```python
from build123d import *
from OCP.BRepFilletAPI import BRepFilletAPI_MakeChamfer

# Parameters (mm, degrees)
SKETCH_1_W       = 40.5
SKETCH_1_H       = 19.8
BODY_DEPTH       = 36.5
CHAMFER_1_SIZE   = 2.2
CHAMFER_1_SIZE2  = 1.4
FILLET_1_R       = 0.5
MOUNT_DEPTH      = 2.5
FILLET_3_R       = 1
EXTRUDE_3_DEPTH  = 0.5
EXTRUDE_4_DEPTH  = 2
SKETCH_5_W       = 10.8
SKETCH_5_H       = 15.84
EXTRUDE_5_DEPTH  = 0.2
SKETCH_6_R       = 6.6
EXTRUDE_6_DEPTH  = 1.2
SKETCH_7_R       = 5.35
EXTRUDE_7_DEPTH  = 0.5
SKETCH_8_R       = 2.6
SHAFT_HOLE_DEPTH = 10
FILLET_2_R       = 0.5
SKETCH_11_R      = 0.75
EXTRUDE_10_DEPTH = 8


with BuildPart() as part:
    # Эскиз1 → Body (new body)
    with BuildSketch(Plane(origin=(0, 0, 0), x_dir=(1, 0, 0), z_dir=(0, 1, 0))):
        Rectangle(SKETCH_1_W, SKETCH_1_H)
    extrude(amount=BODY_DEPTH)

    # Фаска1: one chamfer whose edges measure the first distance from different faces: ONE call of the kernel's chamfer builder (chamfer() names one face for all edges)
    chamfer_1_edges_1 = [part.edges().sort_by_distance(p)[0] for p in [
        (20.25, 36.5, 0),
    ]]
    chamfer_1_side_1 = [part.faces().sort_by_distance(p)[0] for p in [
        (20.25, 18.25, 0),
    ]]
    chamfer_1_edges_2 = [part.edges().sort_by_distance(p)[0] for p in [
        (0, 36.5, -9.9),
    ]]
    chamfer_1_side_2 = [part.faces().sort_by_distance(p)[0] for p in [
        (0, 18.25, -9.9),
    ]]
    chamfer_1_edges_3 = [part.edges().sort_by_distance(p)[0] for p in [
        (-20.25, 36.5, 0),
    ]]
    chamfer_1_side_3 = [part.faces().sort_by_distance(p)[0] for p in [
        (-20.25, 18.25, 0),
    ]]
    chamfer_1_edges_4 = [part.edges().sort_by_distance(p)[0] for p in [
        (0, 36.5, 9.9),
    ]]
    chamfer_1_side_4 = [part.faces().sort_by_distance(p)[0] for p in [
        (0, 18.25, 9.9),
    ]]
    chamfer_1 = BRepFilletAPI_MakeChamfer(part.part.solid().wrapped)
    for e in chamfer_1_edges_1:
        chamfer_1.Add(CHAMFER_1_SIZE, CHAMFER_1_SIZE2, e.wrapped, chamfer_1_side_1[0].wrapped)  # the first distance lies on this face
    for e in chamfer_1_edges_2:
        chamfer_1.Add(CHAMFER_1_SIZE, CHAMFER_1_SIZE2, e.wrapped, chamfer_1_side_2[0].wrapped)  # the first distance lies on this face
    for e in chamfer_1_edges_3:
        chamfer_1.Add(CHAMFER_1_SIZE, CHAMFER_1_SIZE2, e.wrapped, chamfer_1_side_3[0].wrapped)  # the first distance lies on this face
    for e in chamfer_1_edges_4:
        chamfer_1.Add(CHAMFER_1_SIZE, CHAMFER_1_SIZE2, e.wrapped, chamfer_1_side_4[0].wrapped)  # the first distance lies on this face
    add(Compound.cast(chamfer_1.Shape()), mode=Mode.REPLACE)

    # Скругление1
    # the kernel refuses this fillet: 0.5 mm, written as the material it takes off along each edge
    with BuildSketch(Plane(origin=(-20.25, -1.25, 9.9), x_dir=(1, 0, 0), z_dir=(0, 1, 0)), Plane(origin=(-20.25, -1.25, -9.9), x_dir=(0, 0, 1), z_dir=(0, 1, 0))) as fillet_1_piece_1:
        with BuildLine():
            CenterArc((FILLET_1_R, FILLET_1_R), FILLET_1_R, 180, 90)
            Line((0, FILLET_1_R), (0, 0))
            Line((0, 0), (FILLET_1_R, 0))
        make_face()
    extrude(amount=36.8, mode=Mode.SUBTRACT)
    with BuildSketch(Plane(origin=(20.25, -1.25, -9.9), x_dir=(0, 0, 1), z_dir=(0, 1, 0)), Plane(origin=(20.25, -1.25, 9.9), x_dir=(-1, 0, 0), z_dir=(0, 1, 0))) as fillet_1_piece_2:
        with BuildLine():
            CenterArc((FILLET_1_R, -FILLET_1_R), FILLET_1_R, 90, 90)
            Line((0, -FILLET_1_R), (0, 0))
            Line((0, 0), (FILLET_1_R, 0))
        make_face()
    extrude(amount=36.8, mode=Mode.SUBTRACT)
    with BuildSketch(Plane(origin=(20.689497717, 33.609360731, -10.339497717), x_dir=(0.25395078633508533, -0.3990655213836877, 0.8810537485094523), z_dir=(-0.47301616487963943, 0.7433111162394352, 0.47301616487964004)), Plane(origin=(20.689497717, 33.609360731, 10.339497717), x_dir=(-0.8810537485094526, -0.39906552138369156, 0.25395078633507817), z_dir=(-0.47301616487963943, 0.7433111162394352, -0.47301616487964004))) as fillet_1_piece_3:
        with BuildLine():
            CenterArc((FILLET_1_R * 0.743311116239, -FILLET_1_R), FILLET_1_R, 90, 73.247664886)
            Line((-FILLET_1_R * 0.21424849821, -FILLET_1_R * 0.711764705882), (0, 0))
            Line((0, 0), (FILLET_1_R * 0.743311116239, 0))
        make_face()
    extrude(amount=4.818007508, mode=Mode.SUBTRACT)
    with BuildSketch(Plane(origin=(-20.689497717, 33.609360731, -10.339497717), x_dir=(-0.25395078633507856, -0.3990655213836921, 0.8810537485094524), z_dir=(0.47301616487963943, 0.7433111162394352, 0.47301616487964004)), Plane(origin=(-20.689497717, 33.609360731, 10.339497717), x_dir=(0.8810537485094527, -0.3990655213836916, 0.25395078633507817), z_dir=(0.47301616487963943, 0.7433111162394352, -0.47301616487964004))) as fillet_1_piece_4:
        with BuildLine():
            CenterArc((FILLET_1_R * 0.743311116239, FILLET_1_R), FILLET_1_R, 196.752335114, 73.247664886)
            Line((-FILLET_1_R * 0.21424849821, FILLET_1_R * 0.711764705882), (0, 0))
            Line((0, 0), (FILLET_1_R * 0.743311116239, 0))
        make_face()
    extrude(amount=4.818007508, mode=Mode.SUBTRACT)

    # Эскиз2 → Mount (add)
    with BuildSketch(Plane(origin=(0, 6.2, 0), x_dir=(-1, 0, 0), z_dir=(0, -1, 0))):
        with BuildLine():
            Line((-26.85, 9.472835762), (26.85, 9.472835762))
            Line((26.85, 9.472835762), (26.85, 6.069767442))
            Line((26.85, 6.069767442), (26.229418506, 6.069767442))
            ThreePointArc((26.229418506, 6.069767442), (22, 5), (26.229418506, 3.930232558))
            Line((26.229418506, 3.930232558), (26.85, 3.930232558))
            Line((26.85, 3.930232558), (26.85, -3.930232558))
            Line((26.85, -3.930232558), (26.229418506, -3.930232558))
            ThreePointArc((26.229418506, -3.930232558), (22, -5), (26.229418506, -6.069767442))
            Line((26.229418506, -6.069767442), (26.85, -6.069767442))
            Line((26.85, -6.069767442), (26.85, -9.4))
            Line((26.85, -9.4), (-26.85, -9.4))
            Line((-26.85, -9.4), (-26.85, -6.069767442))
            Line((-26.85, -6.069767442), (-26.229418506, -6.069767442))
            ThreePointArc((-26.229418506, -6.069767442), (-22, -5), (-26.229418506, -3.930232558))
            Line((-26.229418506, -3.930232558), (-26.85, -3.930232558))
            Line((-26.85, -3.930232558), (-26.85, 3.930232558))
            Line((-26.85, 3.930232558), (-26.229418506, 3.930232558))
            ThreePointArc((-26.229418506, 3.930232558), (-22, 5), (-26.229418506, 6.069767442))
            Line((-26.229418506, 6.069767442), (-26.85, 6.069767442))
            Line((-26.85, 6.069767442), (-26.85, 9.472835762))
        make_face()
    extrude(amount=-MOUNT_DEPTH)

    # Скругление3
    fillet_3_edges = [part.edges().sort_by_distance(p)[0] for p in [
        (-26.85, 7.45, 9.4),
        (26.85, 7.45, 9.4),
        (26.85, 7.45, -9.472835762),
        (-26.85, 7.45, -9.472835762),
    ]]
    fillet(fillet_3_edges, radius=FILLET_3_R)

    # Эскиз3 → Бобышка-Вытянуть3 (add, symmetric)
    with BuildSketch(Plane.XY):
        Polygon((-26.85, 6.2), (-20.25, 6.2), (-20.25, 5.2), align=None)
        Polygon((20.25, 5.2), (26.85, 6.2), (20.25, 6.2), align=None)
    extrude(amount=EXTRUDE_3_DEPTH, both=True)

    # Эскиз4 → Бобышка-Вытянуть4 (add)
    with BuildSketch(Plane.XZ):
        with BuildLine():
            Line((-13.452560024, -8.92), (-13.452560024, -4.6))
            ThreePointArc((-13.452560024, -4.6), (-16.49296823, 0), (-13.452560024, 4.6))
            Line((-13.452560024, 4.6), (-13.452560024, 8.92))
            Line((-13.452560024, 8.92), (6.568139057, 8.92))
            ThreePointArc((6.568139057, 8.92), (19.9, 0), (6.568139057, -8.92))
            Line((6.568139057, -8.92), (-13.452560024, -8.92))
        make_face()
    extrude(amount=EXTRUDE_4_DEPTH)

    # Эскиз5 → Бобышка-Вытянуть5 (add)
    with BuildSketch(Plane.XZ.offset(2)):
        with BuildLine():
            Line((-13.452560024, 8.92), (-0.652560024, 8.92))
            Line((-0.652560024, 8.92), (-0.652560024, 2))
            ThreePointArc((-0.652560024, 2), (1.347439976, 0), (-0.652560024, -2))
            Line((-0.652560024, -2), (-0.652560024, -8.92))
            Line((-0.652560024, -8.92), (-13.452560024, -8.92))
            Line((-13.452560024, -8.92), (-13.452560024, 8.92))
        make_face()
        with Locations((-7.052560024, 0)):
            Rectangle(SKETCH_5_W, SKETCH_5_H, mode=Mode.SUBTRACT)
    extrude(amount=EXTRUDE_5_DEPTH)

    # Эскиз6 → Бобышка-Вытянуть6 (add)
    with BuildSketch(Plane.XZ.offset(2)):
        with Locations(Location((10.25, 0, 0), (0, 0, 270))):
            Circle(SKETCH_6_R)
    extrude(amount=EXTRUDE_6_DEPTH)

    # Эскиз7 → Бобышка-Вытянуть7 (add)
    with BuildSketch(Plane.XZ.offset(3.2)):
        with Locations(Location((10.25, 0, 0), (0, 0, 270))):
            Circle(SKETCH_7_R)
    extrude(amount=EXTRUDE_7_DEPTH)

    # Эскиз8 → Shaft hole (cut)
    with BuildSketch(Plane.XZ.offset(3.7)):
        with Locations(Location((10.25, 0, 0), (0, 0, 270))):
            Circle(SKETCH_8_R)
    extrude(amount=-SHAFT_HOLE_DEPTH, mode=Mode.SUBTRACT)

    # Скругление2
    fillet_2_edges = [part.edges().sort_by_distance(p)[0] for p in [
        (-13.452560024, -1.1, 8.92),
        (-0.652560024, -2.1, 2),
        (-0.652560024, -2.1, -2),
        (-0.652560024, -2.1, 8.92),
        (-0.652560024, -2.1, -8.92),
        (-13.452560024, -1.1, -8.92),
        (-1.652560024, -2.1, 7.92),
        (-1.652560024, -2.1, -7.92),
        (-12.452560024, -2.1, 7.92),
        (-12.452560024, -2.1, -7.92),
    ]]
    fillet(fillet_2_edges, radius=FILLET_2_R)

    # Эскиз10 → Rubber section 0
    with BuildSketch(Plane(origin=(25.25, 0, 0), x_dir=(0, 0, -1), z_dir=(1, 0, 0))):
        with BuildLine():
            Line((-2.5, 29.75), (2.5, 29.75))
            Line((2.5, 29.75), (2.5, 32.55))
            Line((2.5, 32.55), (-2.5, 32.55))
            Line((-2.5, 32.55), (-2.5, 29.75))
        make_face()
    # Эскиз9 → Rubber section 1
    with BuildSketch(Plane(origin=(20.25, 0, 0), x_dir=(0, 0, -1), z_dir=(1, 0, 0))):
        with BuildLine():
            Line((-3.4, 33.3), (3.4, 33.3))
            Line((3.4, 33.3), (3.4, 29))
            Line((3.4, 29), (-3.4, 29))
            Line((-3.4, 29), (-3.4, 33.3))
        make_face()
    loft()

    # Эскиз11 → Бобышка-Вытянуть10 (add)
    with BuildSketch(Plane(origin=(25.25, 0, 0), x_dir=(0, 0, -1), z_dir=(1, 0, 0))):
        with Locations(Location((0, 31.150503064, 0), (0, 0, 180))):
            Circle(SKETCH_11_R)
        with Locations(Location((1.509999917, 31.15000331, 0), (0, 0, 180))):
            Circle(SKETCH_11_R)
        with Locations(Location((-1.509999915, 31.149996646, 0), (0, 0, 180))):
            Circle(SKETCH_11_R)
    extrude(amount=EXTRUDE_10_DEPTH)


solid = part.part
```
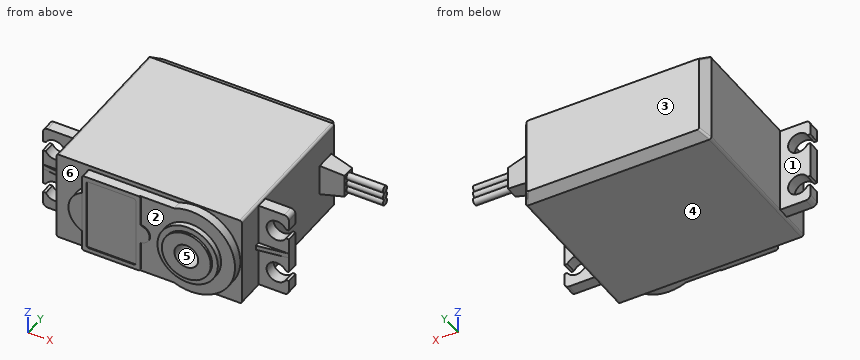
CAD build for the part. Positions are in the model's coordinates, mm. Face numbers are marked on the shaded views. A direction names the side the tool comes from. Coordinates: 2 decimals unless noted, no trailing zeros. Loops run counter-clockwise (first coordinate to the right, second up) from the corner with the lowest first, then second, coordinate; pieces in that order, holes last. Notation, with made-up numbers: (53, 37) - (98, 37) arc R24 ccw to (98, 76) - close; hole circle Ø4 at (24, 14.5). An arc over 180 degrees is marked (long way). Return JSON: item names as keys, results as strings.
1. Band-saw the part on D-D (y = 16). Give the cut face in (x, z).
Result:
{"outline": "(-20.25, -9.4) arc R0.5 ccw to (-19.75, -9.9) - (19.75, -9.9) arc R0.5 ccw to (20.25, -9.4) - (20.25, 9.4) arc R0.5 ccw to (19.75, 9.9) - (-19.75, 9.9) arc R0.5 ccw to (-20.25, 9.4) - close"}
2. Band-saw the part on A-A (x = -24.25). Give the cut face in (y, z), and give its area (3 significant figures).
Result:
{"outline": "(5.81, -0.5) - (6.2, -0.5) - (6.2, -2.75) - (8.7, -2.75) - (8.7, 2.75) - (6.2, 2.75) - (6.2, 0.5) - (5.81, 0.5) - close; (6.2, -9.47) - (8.7, -9.47) - (8.7, -7.25) - (6.2, -7.25) - close; (6.2, 7.25) - (8.7, 7.25) - (8.7, 9.4) - (6.2, 9.4) - close", "area": "25.1 mm2"}
3. 3-axis set-ups, long thin cutter, end or side, ignore diameter. For the marked faces 1, 2 and 3: which of +Z, -Z, +X, -X, +Y, -Y reach the whole face in a straight line?
Result:
{"face 1": "+Z, -Z, -X, +Y", "face 2": "-Y", "face 3": "+Z, -Z, +X, -X, +Y"}
4. Drop flat-ended pins along their axis: pin 1 (0.7 mm diameter, centred on x = -23.5, y = 7, fed in from -Z); pin 2 (8 mm diameter, centred on x = -16, z = -0.5, fed in from -Y); pin 3 (0.5 mm diameter, centred on x = -26.5, y = 8, fed in from -Z). Give the stop position or say it passes through.
Result:
{"pin 1": "stops at z = -9.47", "pin 2": "stops at y = -2.2", "pin 3": "stops at z = -9.39"}
5. Band-saw the part on C-C (x = 10.25). Give the cut face in (y, z).
Result:
{"outline": "(-3.7, -5.35) - (-3.2, -5.35) - (-3.2, -6.6) - (-2, -6.6) - (-2, -9.65) - (0, -9.65) - (0, -9.9) - (34.3, -9.9) - (36.5, -8.5) - (36.5, 8.5) - (34.3, 9.9) - (0, 9.9) - (0, 9.65) - (-2, 9.65) - (-2, 6.6) - (-3.2, 6.6) - (-3.2, 5.35) - (-3.7, 5.35) - (-3.7, 2.6) - (6.3, 2.6) - (6.3, -2.6) - (-3.7, -2.6) - close"}
6. Probe L1, parallel to Z at x = -24.25, y = 6.95; L2, parallel to X at y = 0.5, z = 0; L3, parallel to X at y = 17, z = -1. List the from-to ranges inside material, lowest first. Write a range as from..to.
Result:
{"L1": "z = -9.47..-7.25, -2.75..2.75, 7.25..9.4", "L2": "x = -20.25..7.65, 12.85..20.25", "L3": "x = -20.25..20.25"}
7. Mould opens along Z. For the marked faces 4, 5 and 6 say: released by +Z, released by -Z, zero draft, split by the parting line, or undercut.
Result:
{"face 4": "released by -Z", "face 5": "undercut", "face 6": "zero draft"}
